```python
from build123d import *

# Parameters (mm, degrees)
SKETCH1_W           = 20
SKETCH1_H           = 8
BOSS_EXTRUDE1_DEPTH = 8
SKETCH2_R           = 1.4
CUT_EXTRUDE1_DEPTH  = 7
CUT_EXTRUDE2_DEPTH  = 5
CUT_EXTRUDE3_DEPTH  = 2.5


with BuildPart() as part:
    # Sketch1 → Boss-Extrude1 (new body)
    with BuildSketch(Plane(origin=(0, 0, 0), x_dir=(1, 0, 0), z_dir=(0, 1, 0))):
        with Locations((10, 4)):
            Rectangle(SKETCH1_W, SKETCH1_H)
    extrude(amount=BOSS_EXTRUDE1_DEPTH)

    # Sketch2 → Cut-Extrude1 (cut)
    with BuildSketch(Plane(origin=(0, 8, 0), x_dir=(1, 0, 0), z_dir=(0, 1, 0))):
        with BuildLine():
            Line((20, 6.5), (10, 6.5))
            ThreePointArc((10, 6.5), (7.2, 3.7), (10, 0.9))
            Line((10, 0.9), (12, 0.9))
            ThreePointArc((12, 0.9), (12.707106781, 1.192893219), (13, 1.9))
            Line((13, 1.9), (13, 3.5))
            ThreePointArc((13, 3.5), (13.292893219, 4.207106781), (14, 4.5))
            Line((14, 4.5), (20, 4.5))
            Line((20, 4.5), (20, 6.5))
        make_face()
        with Locations(Location((10, 3.7, 0), (0, 0, 270))):
            Circle(SKETCH2_R, mode=Mode.SUBTRACT)
    extrude(amount=-CUT_EXTRUDE1_DEPTH, mode=Mode.SUBTRACT)

    # Sketch4 → Cut-Extrude2 (cut)
    with BuildSketch(Plane.ZY):
        with BuildLine():
            Line((-5.75, 4), (-5.75, 8))
            Line((-5.75, 8), (-2.25, 8))
            Line((-2.25, 8), (-2.25, 4))
            ThreePointArc((-2.25, 4), (-4, 2.25), (-5.75, 4))
        make_face()
    extrude(amount=-CUT_EXTRUDE2_DEPTH, mode=Mode.SUBTRACT)

    # Sketch5 → Cut-Extrude3 (cut)
    with BuildSketch(Plane.ZY.offset(-5)):
        Polygon((-7.175426481, 3.5), (-7.175426481, 14.06619177), (-1.206769201, 14.06619177), (-1.206769201, 3.638089636), (-1.953153528, 1.572294735), (-5.079031196, 1.013526325), align=None)
    extrude(amount=CUT_EXTRUDE3_DEPTH, mode=Mode.SUBTRACT)


solid = part.part
```
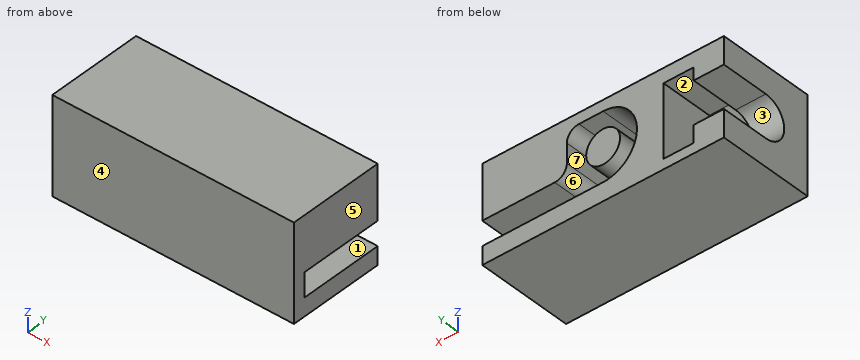
Verification items for the finished model (mm, model axes). Face numbers are marked on the shaded views. A direction names the side the tool comes from. Coordinates: 2 decimals unless noted, no trailing zeros. Write each loop counter-clockwise with the first axis right and the second up, starting at its lowest first coordinate (ties: lowest second). Pieces come first, ordered by that corner, then holes. Notation, with made-up numbers: (8, 77.5) - (63, 77.5) arc R13 ccw to (63, 94.5) - close; hole circle Ø1 at (82, 2). An arc over 180 degrees is marked (long way). Write item = value, one per line.
Q1. Cross-section at C-C (y = 2). Enter the section's corners in (x, z).
Answer:
outline = (0, -8) - (20, -8) - (20, -6.5) - (10, -6.5) arc R2.8 cw to (10, -0.9) - (12, -0.9) arc R1 cw to (13, -1.9) - (13, -3.5) arc R1 ccw to (14, -4.5) - (20, -4.5) - (20, 0) - (0, 0) - close; circle Ø2.8 at (10, -3.7); hole (2.5, -5.91) - (5, -5.91) - (5, -1.8) - (2.5, -1.8) - close
Q2. Go/stop test with flat-tipped pins: pin 1 Ø1 at (x, z) = (3.5, -6.5) entering from +Y; pin 2 Ø0.8 at (y, z) = (5, -3) entering from -X. Record where each tip stops, or that it passes through.
Answer:
pin_1 = 3.29
pin_2 = 5
Q3. Mould release check, pull along X, two halves, no side actions. Record for the marked faces 4, 5, 6 and 7: released by +X, released by -X, zero draft, split by the parting line, or undercut.
Answer:
face_4 = zero draft
face_5 = released by +X
face_6 = undercut
face_7 = undercut
Q4. Cross-section at B-B (x = 4.75). Enter the section's corners in (y, z).
Answer:
outline = (0, -8) - (8, -8) - (8, -7.18) - (3.5, -7.18) - (1.01, -5.08) - (1.57, -1.95) - (3.64, -1.21) - (8, -1.21) - (8, 0) - (0, 0) - close
Q5. Cross-section at A-A (y = 5.5). Enter the section's corners in (x, z), plus the area to 3 significant figures.
Answer:
outline = (0, -8) - (20, -8) - (20, -6.5) - (10, -6.5) arc R2.8 cw to (10, -0.9) - (12, -0.9) arc R1 cw to (13, -1.9) - (13, -3.5) arc R1 ccw to (14, -4.5) - (20, -4.5) - (20, 0) - (0, 0) - (0, -2.25) - (2.5, -2.25) - (2.5, -1.21) - (5, -1.21) - (5, -7.18) - (2.5, -7.18) - (2.5, -5.75) - (0, -5.75) - close; circle Ø2.8 at (10, -3.7)
area = 99.4 mm²
Q6. Access from +Z, -Z, +X, -X, +Y, -Y to the whole of each face (thin tool, end or side, straight path). Record for the marked faces 1, 2 and 3.
Answer:
face_1 = +X, +Y
face_2 = +Y
face_3 = -X, +Y
Q7. Material ranges on L1, parallel to X at y = 7.5, z = -6.75; L2, parallel to X at y = 6.5, z = -1.5; L3, parallel to Z at x = 4, y = 5.5, recorded low to high. Write a range as from..to.
Answer:
L1 = 0..2.5, 5..20
L2 = 0..2.5, 5..8.27, 12.92..20
L3 = -8..-7.18, -1.21..0
Q8. Cross-section at D-D (z = -4). Enter the section's corners in (x, y).
Answer:
outline = (0, 0) - (20, 0) - (20, 8) - (13.13, 8) - (13.13, 1) - (11.37, 1) - (11.37, 8) - (8.63, 8) - (8.63, 1) - (7.22, 1) - (7.22, 8) - (5, 8) - (5, 1.21) - (2.5, 1.21) - (2.5, 2.25) - (0, 2.25) - close
